Source: CAD feature listing. Evaluate the final solid. Frame: model axes, mm. A direction names the side the tool comes from. Coordinates: 2 decimals unless noted, no trailing zeros. Write each loop counter-clockwise with the first axis right and the second up, starting at its lowest first coordinate (ties: lowest second). Pieces come first, ordered by that corner, then holes. Notation, with made-up numbers: M 22,-13 L 75,-13 A34 cw 75,26 Z; hole C -40,24.5 d9. An arc over 180 degrees is marked long. Write item = value, one per line. Start each with the question number.
1. Line query: line 1 along X through (y, z) = (5, 0); line 2 along Z through (x, y) = (-13.5, 4); line 3 along X through (y, z) = (3.5, 24.5). Output: solid intervals per line, ascending.
2. Pin query (flat end, axial travel): pin 1 Ø1 at (x, z) = (11.5, -14) entering from +Y; pin 2 Ø1 at (y, z) = (2, 20.5) entering from +X; pin 3 Ø2 at (x, z) = (13.5, 23.38) entering from -Y (1 decimal); pin 4 Ø4 at (y, z) = (5, -4.5) entering from +X. Return the tip coordinate at first contact, or that it passes through.
3. Section query C-C (z = 19). Output: boundary loops of the cut face in (x, y), then the cut area to 3 significant figures.
4. Section query B-B (y = 6). Give the number of separate pieces and of enclosed holes in the cut face, then the cut area to 3 significant figures.
5. Access query for faces 1 (the face through (-12, 2.3, 0)), 2 (the face through (13.28, 4.14, -25.07)). Directions: +Z, -Z, +X, -X, +Y, -Y. A direction counts if a zero-diameter tool reaches every point of the face in a straight line with its end or side. Return the directions, or none.
6. Section query D-D (x = 13.5). Output: boundary loops of the cut face in (y, z).
7. Section query A-A (x = 0). Output: boundary loops of the cut face in (y, z).
```python
from build123d import *

# Parameters (mm, degrees)
M3_CLEARANCE_HOLE1_OUTLINE_R = 1.7
M3_CLEARANCE_HOLE1_DEPTH     = 8.4
CHAMFER1_SIZE                = 0.4


# Read off the part's stored shape, not the designer's step: M3 Clearance Hole1
with BuildPart() as part:
    # Sketch1 → Revolve1 (revolve)
    with BuildSketch(Plane.XY, mode=Mode.PRIVATE) as revolve1_sk:
        Polygon((2.7, 0), (2.7, 8.4), (4.1, 8.4), (4.1, 3.3), (11.5, 3.3), (11.5, 2.3), (15.5, 2.3), (15.5, 3.3), (22.1, 3.3), (22.1, 8.4), (30, 8.4), (30, 0), align=None)
    revolve(revolve1_sk.sketch.rotate(Axis((0, 16.309231771, 0), (0, -1, 0)), 90), axis=Axis((0, 16.309231771, 0), (0, -1, 0)))

    # M3 Clearance Hole1 outline → M3 Clearance Hole1 (cut)
    with BuildSketch(Plane(origin=(0, 0, 0), x_dir=(1, 0, 0), z_dir=(0, 1, 0))):
        with Locations((13.5, -23.382685902)):
            Circle(M3_CLEARANCE_HOLE1_OUTLINE_R)
        with Locations((-13.5, -23.382685902)):
            Circle(M3_CLEARANCE_HOLE1_OUTLINE_R)
        with Locations((-27, 0)):
            Circle(M3_CLEARANCE_HOLE1_OUTLINE_R)
        with Locations((-13.5, 23.382685902)):
            Circle(M3_CLEARANCE_HOLE1_OUTLINE_R)
        with Locations((13.5, 23.382685902)):
            Circle(M3_CLEARANCE_HOLE1_OUTLINE_R)
        with Locations((27, 0)):
            Circle(M3_CLEARANCE_HOLE1_OUTLINE_R)
    extrude(amount=M3_CLEARANCE_HOLE1_DEPTH, mode=Mode.SUBTRACT)

    # Chamfer1
    chamfer1_edges = [part.edges().sort_by_distance(p)[0] for p in [
        (0, 3.3, -4.1),
    ]]
    chamfer(chamfer1_edges, length=CHAMFER1_SIZE)


solid = part.part
```
Results are:
q1.line_1 = -30 to -28.7, -25.3 to -22.1, -4.1 to -2.7, 2.7 to 4.1, 22.1 to 25.3, 28.7 to 30
q1.line_2 = -26.79 to -25.08, -21.68 to -17.5, 17.5 to 21.68, 25.08 to 26.79
q1.line_3 = -17.31 to -14.78, -12.22 to 12.22, 14.78 to 17.31
q2.pin_1 = 3.3
q2.pin_2 = 22.36
q2.pin_3 = through
q2.pin_4 = 29.9
q3.outline = M -23.22,0 L 23.22,0 L 23.22,8.4 L 11.29,8.4 L 11.29,3.3 L -11.29,3.3 L -11.29,8.4 L -23.22,8.4 Z
q3.area = 275 mm^2
q4.separate_pieces = 2
q4.enclosed_holes = 8
q4.area = 1,270 mm^2
q5.face_1 = +Y
q5.face_2 = +Y, -Y
q6.outline = M 0,-26.79 L 8.4,-26.79 L 8.4,-25.08 L 0,-25.08 Z; M 0,-21.68 L 8.4,-21.68 L 8.4,-17.5 L 3.3,-17.5 L 3.3,-7.62 L 2.3,-7.62 L 2.3,7.62 L 3.3,7.62 L 3.3,17.5 L 8.4,17.5 L 8.4,21.68 L 0,21.68 Z; M 0,25.08 L 8.4,25.08 L 8.4,26.79 L 0,26.79 Z
q7.outline = M 0,-30 L 8.4,-30 L 8.4,-22.1 L 3.3,-22.1 L 3.3,-15.5 L 2.3,-15.5 L 2.3,-11.5 L 3.3,-11.5 L 3.3,-4.5 L 3.7,-4.1 L 8.4,-4.1 L 8.4,-2.7 L 0,-2.7 Z; M 0,2.7 L 8.4,2.7 L 8.4,4.1 L 3.7,4.1 L 3.3,4.5 L 3.3,11.5 L 2.3,11.5 L 2.3,15.5 L 3.3,15.5 L 3.3,22.1 L 8.4,22.1 L 8.4,30 L 0,30 Z
